```python
from build123d import *

# Parameters (mm, degrees)
F1_DEPTH = 3.5
F2_R     = 1.8
F3_DEPTH = 8
F4_R     = 1.8
F5_DEPTH = 8000


with BuildPart() as f1:
    # F0 (on Top) → F1 (new body, symmetric)
    with BuildSketch(Plane.XY):
        with BuildLine():
            ThreePointArc((50, 5), (45.606602, 15.606602), (35, 20))
            Line((35, 20), (-35, 20))
            ThreePointArc((-35, 20), (-45.606602, 15.606602), (-50, 5))
            Line((-50, 5), (-50, -5))
            ThreePointArc((-50, -5), (-45.606602, -15.606602), (-35, -20))
            Line((-35, -20), (35, -20))
            ThreePointArc((35, -20), (45.606602, -15.606602), (50, -5))
            Line((50, -5), (50, 5))
        make_face()
    extrude(amount=F1_DEPTH, both=True)

    # F2 (on face) → F3 (cut)
    with BuildSketch(Plane.XY.offset(3.5)):
        with Locations((-35, 5)):
            Circle(F2_R)
        with Locations((-35, -5)):
            Circle(F2_R)
    extrude(amount=-F3_DEPTH, mode=Mode.SUBTRACT)

    # F4 (on face) → F5 (cut)
    with BuildSketch(Plane.XY.offset(3.5)):
        with Locations((41.754141, 0)):
            Circle(F4_R)
    extrude(amount=-F5_DEPTH, mode=Mode.SUBTRACT)


solid = f1.part
```
CAD build for the part. Positions are in the model's coordinates, mm. Give positions to 0.01 mm unless a question says otherwise; leave off trailing zeros. Order: outer loops, then holes, each group sorted by start corner. A loop starts at its lowest first (then second) coordinate and runs counter-clockwise, first axis right, second up.
(1) Saw through at B-B, the plane z = 2. Give the cut face in (x, y).
(2) Drill centre lines: L1, parallel to Y at x = -35, z = -1.25; L2, parallel to Y at x = 35.5, z = 3.25; L3, parallel to X at y = 3.5, z = 3. Where is each one in solid material? Low to high.
(3) Saw through at D-D, the plane y = 14.5. Give the cut face in (x, z), then the cut area to 3 significant figures.
(4) Mould opens along X. For faces 1 (the cylindrical face through (45.72, 15.49, 0.05)), 2 (the flat face through (-1, 0, 3.5)), 3 (the cylindrical face through (-33.283, -4.459, 0.049)) say: released by +X, released by -X, zero draft, split by the parting line, or undercut.
(5) Saw through at C-C, the plane x = -40. Give the cut face in (y, z), then the cut area to 3 significant figures.
(6) Saw through at A-A, the plane y = 0. Give the cut face in (x, z).
(7) Flat gauge pins, fed straight in: pin 1 (3 mm diameter, centred on x = -35, y = -5, fed in from +Z); pin 2 (1 mm diameter, centred on y = -10, z = -0.5, fed in from +X). Where does each tip first touch, or does it go through?
Results found:
1. outline: (-50, -5) arc R15 ccw to (-35, -20) - (35, -20) arc R15 ccw to (50, -5) - (50, 5) arc R15 ccw to (35, 20) - (-35, 20) arc R15 ccw to (-50, 5) - close; hole circle Ø3.6 at (-35, -5); hole circle Ø3.6 at (-35, 5); hole circle Ø3.6 at (41.75, 0)
2. L1: y = -20 to -6.8, -3.2 to 3.2, 6.8 to 20
2. L2: y = -19.99 to 19.99
2. L3: x = -50 to -35.99, -34.01 to 50
3. outline: (-46.61, -3.5) - (46.61, -3.5) - (46.61, 3.5) - (-46.61, 3.5) - close
3. area: 653 mm2
4. face 1: released by +X
4. face 2: zero draft
4. face 3: undercut
5. outline: (-19.14, -3.5) - (19.14, -3.5) - (19.14, 3.5) - (-19.14, 3.5) - close
5. area: 268 mm2
6. outline: (-50, -3.5) - (39.95, -3.5) - (39.95, 3.5) - (-50, 3.5) - close; (43.55, -3.5) - (50, -3.5) - (50, 3.5) - (43.55, 3.5) - close
7. pin 1: passes through
7. pin 2: stops at x = 49.31
